Verification items for the finished model (mm, model axes). Round coordinates to 2 decimals unless told otherwise and drop trailing zeros. Order: outer loops, then holes, each group sorted by start corner. A loop starts at its lowest first (then second) coordinate and runs counter-clockwise, first axis right, second up. Notation, with made-up numbers: (39, 25) -> (94, 25) arc R21 cw to (94, 33) -> close; hole circle Ø5 at (61, 55). An arc over 180 degrees is marked (long way). Put each result on its own line as item: value.
```python
from build123d import *

# Parameters (mm, degrees)
BOSS_EXTRUDE1_DEPTH = 900
FILLET1_START       = -1
FILLET1_DEPTH       = 2052


with BuildPart() as part:
    # Sketch1 → Boss-Extrude1 (new body)
    with BuildSketch(Plane(origin=(0, 0, 0), x_dir=(1, 0, 0), z_dir=(0, 1, 0))):
        with BuildLine():
            Line((0, 0), (10.739185416, 0))
            ThreePointArc((10.739185416, 0), (1025, 690.782014433), (2039.260814584, 0))
            Line((2039.260814584, 0), (2050, 0))
            ThreePointArc((2050, 0), (1025, 700.782014433), (0, 0))
        make_face()
    extrude(amount=BOSS_EXTRUDE1_DEPTH)

    # Fillet1: read off the stored shape, not the designer's step
    # Fillet1 outline → Fillet1 (cut)
    with BuildSketch(Plane.YZ.offset(FILLET1_START)):
        with BuildLine():
            ThreePointArc((0, -100), (29.289321881, -29.289321881), (100, 0))
            Line((100, 0), (0, 0))
            Line((0, 0), (0, -100))
        make_face()
        with BuildLine():
            ThreePointArc((800, 0), (870.710678119, -29.289321881), (900, -100))
            Line((900, -100), (900, 0))
            Line((900, 0), (800, 0))
        make_face()
    extrude(amount=FILLET1_DEPTH, mode=Mode.SUBTRACT)


solid = part.part
```
Item 1: Material ranges on line 1 along X through (y, z) = (180, -364); line 2 along X through (y, z) = (409, -573); line 3 along Z through (x, y) = (1052.5, 266), recorded low to high.
Geometry check:
line 1: 232.85 to 246.8, 1803.2 to 1817.15
line 2: 510.42 to 532.16, 1517.84 to 1539.58
line 3: -700.44 to -690.44
Item 2: Release check for a two-part mould opening along X. For faces 1 (the face through (1006.75, 443.7, -690.63)), 2 (the face through (1043.47, 443.7, -700.627)), 3 (the face through (1166, 900, -691)) record: pulls with the +X half, pulls with the -X half, needs draft (parallel to the pull), parting line crosses it, or undercut.
Geometry check:
face 1: undercut
face 2: parting line crosses it
face 3: needs draft
Item 3: Sectioned sample at A-A, the plane z = -582.5. Record the boundary of the cut face in (x, y).
Geometry check:
outline: (528.78, 0) -> (551.37, 0) -> (551.37, 900) -> (528.78, 900) -> close; (1498.63, 0) -> (1521.22, 0) -> (1521.22, 900) -> (1498.63, 900) -> close
Item 4: Depth check by flat-ended pin: pin 1 Ø1 at (x, y) = (451.5, 546) entering from -Z. Enter the tip coordinate at first touch or a pass-through.
Geometry check:
pin 1: z = -539.76
Item 5: Sectioned sample at B-B, the plane y = 650. Record the boundary of the cut face in (x, z).
Geometry check:
outline: (0, 0) arc R1100 ccw to (2050, 0) -> (2039.26, 0) arc R1090 cw to (10.74, 0) -> close
